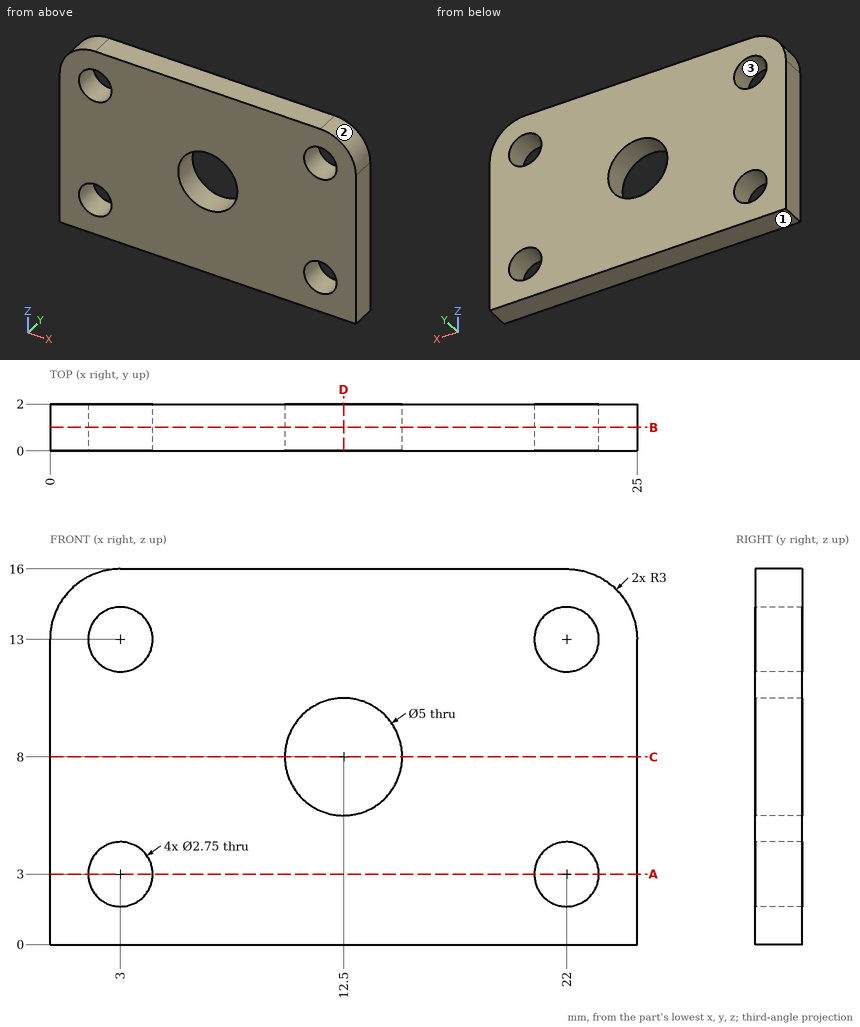
Geometry check sheet. Reference: drawing and pictorial views, mm from the part's lowest x, y, z. Coordinates: 2 decimals unless noted, no trailing zeros. Order: outer loops, then holes, each group sorted by start corner. A loop starts at its lowest first (then second) coordinate and runs counter-clockwise, first axis right, second up.
Item 1: Section check B-B (y = 1). Enter the section's corners in (x, z) (3 decimals), plus the area to 3 significant figures.
Item 2: Section check D-D (x = 12.5). Enter the section's corners in (y, z), plus the area to 3 significant figures.
Item 3: Section check C-C (z = 8). Enter the section's corners in (x, y).
Item 4: Mould release check, pull along X, two halves, no side actions. Record for the marked faces 1, 2 and 3: released by +X, released by -X, zero draft, split by the parting line, or undercut.
Item 5: Scan lines: line 1 along Z through (x, y) = (3, 1.25) (3 decimals); line 2 along X through (y, z) = (0.3, 13.5); line 3 along Z through (x, y) = (3.75, 0.6). Record each from-to range of solid material in increasing order.
Item 6: Section check A-A (z = 3). Enter the section's corners in (x, y) (3 decimals).
Check sheet entries:
1. outline: (0, 0) - (25, 0) - (25, 13) arc R3 ccw to (22, 16) - (3, 16) arc R3 ccw to (0, 13) - close; hole circle Ø2.75 at (3, 3); hole circle Ø2.75 at (3, 13); hole circle Ø5 at (12.5, 8); hole circle Ø2.75 at (22, 3); hole circle Ø2.75 at (22, 13)
1. area: 353 mm2
2. outline: (0, 0) - (2, 0) - (2, 5.5) - (0, 5.5) - close; (0, 10.5) - (2, 10.5) - (2, 16) - (0, 16) - close
2. area: 22.0 mm2
3. outline: (0, 0) - (10, 0) - (10, 2) - (0, 2) - close; (15, 0) - (25, 0) - (25, 2) - (15, 2) - close
4. face 1: zero draft
4. face 2: released by +X
4. face 3: undercut
5. line 1: z = 0 to 1.625, 4.375 to 11.625, 14.375 to 16
5. line 2: x = 0.04 to 1.72, 4.28 to 20.72, 23.28 to 24.96
5. line 3: z = 0 to 1.85, 4.15 to 11.85, 14.15 to 16
6. outline: (0, 0) - (1.625, 0) - (1.625, 2) - (0, 2) - close; (4.375, 0) - (20.625, 0) - (20.625, 2) - (4.375, 2) - close; (23.375, 0) - (25, 0) - (25, 2) - (23.375, 2) - close
